```python
from build123d import *

# Parameters (mm, degrees)
MODEL_R             = 1.775
MODEL_R_2           = 1.575
MODEL_W             = 19.75
MODEL_H             = 93.75
MODEL_W_2           = 17.75
BOSS_EXTRUDE1_DEPTH = 10


with BuildPart() as part:
    # Model → Boss-Extrude1 (new body)
    with BuildSketch(Plane.XY):
        Polygon((57.946480534, -88.339102909), (57.946480534, -68.089102909), (54.771480534, -68.089102909), (54.771480534, -48.339102909), (57.946480534, -48.339102909), (57.946480534, -28.089102909), (54.771480534, -28.089102909), (54.771480534, -8.339102909), (57.946480534, -8.339102909), (57.946480534, 11.910897091), (54.771480534, 11.910897091), (54.771480534, 31.660897091), (57.946480534, 31.660897091), (57.946480534, 51.910897091), (54.771480534, 51.910897091), (54.771480534, 71.660897091), (57.946480534, 71.660897091), (57.946480534, 91.910897091), (54.771480534, 91.910897091), (54.771480534, 111.660897091), (57.946480534, 111.660897091), (57.946480534, 131.910897091), (54.771480534, 131.910897091), (54.771480534, 151.660897091), (57.946480534, 151.660897091), (57.946480534, 161.910897091), (-172.303519466, 161.910897091), (-172.303519466, 151.660897091), (-169.128519466, 151.660897091), (-169.128519466, 131.910897091), (-172.303519466, 131.910897091), (-172.303519466, 111.660897091), (-169.128519466, 111.660897091), (-169.128519466, 91.910897091), (-172.303519466, 91.910897091), (-172.303519466, 71.660897091), (-169.128519466, 71.660897091), (-169.128519466, 51.910897091), (-172.303519466, 51.910897091), (-172.303519466, 31.660897091), (-169.128519466, 31.660897091), (-169.128519466, 11.910897091), (-172.303519466, 11.910897091), (-172.303519466, -8.339102909), (-169.128519466, -8.339102909), (-169.128519466, -28.089102909), (-172.303519466, -28.089102909), (-172.303519466, -48.339102909), (-169.128519466, -48.339102909), (-169.128519466, -68.089102909), (-172.303519466, -68.089102909), (-172.303519466, -88.339102909), align=None)
        with Locations((-12.413986694, 38.429929163)):
            Circle(MODEL_R, mode=Mode.SUBTRACT)
        with Locations((4.096306466, 38.429929163)):
            Circle(MODEL_R_2, mode=Mode.SUBTRACT)
        with Locations((4.008638821, 82.124992621)):
            Circle(MODEL_R_2, mode=Mode.SUBTRACT)
        with Locations((-45.560089874, 82.12499262)):
            Circle(MODEL_R_2, mode=Mode.SUBTRACT)
        with Locations((-45.560089874, 38.429929163)):
            Circle(MODEL_R_2, mode=Mode.SUBTRACT)
        with Locations((-68.972284348, 38.429929163)):
            Circle(MODEL_R_2, mode=Mode.SUBTRACT)
        with Locations((-68.972284348, 82.12499262)):
            Circle(MODEL_R_2, mode=Mode.SUBTRACT)
        with Locations((-102.118387528, 38.429929163)):
            Circle(MODEL_R, mode=Mode.SUBTRACT)
        with Locations((-118.541013043, 38.429929163)):
            Circle(MODEL_R_2, mode=Mode.SUBTRACT)
        with Locations((-118.541013043, 82.12499262)):
            Circle(MODEL_R_2, mode=Mode.SUBTRACT)
        with Locations((-118.541013043, 116.547553094)):
            Circle(MODEL_R_2, mode=Mode.SUBTRACT)
        with Locations((-102.118387528, 128.129929163)):
            Circle(MODEL_R, mode=Mode.SUBTRACT)
        with Locations((-12.413986694, 128.129929163)):
            Circle(MODEL_R, mode=Mode.SUBTRACT)
        with Locations((4.008638821, 116.547553094)):
            Circle(MODEL_R_2, mode=Mode.SUBTRACT)
        with Locations((-142.266187111, 104.785897091)):
            Rectangle(MODEL_W, MODEL_H, mode=Mode.SUBTRACT)
        with Locations((26.821480534, 104.785897091)):
            Rectangle(MODEL_W_2, MODEL_H, mode=Mode.SUBTRACT)
    extrude(amount=BOSS_EXTRUDE1_DEPTH)


solid = part.part
```
Here's how the part is built. I have some questions about the finished solid (model axes, mm). A direction names the side the tool comes from. Round coordinates to 2 decimals unless told otherwise and drop trailing zeros. Loops run counter-clockwise (first coordinate to the right, second up) from the corner with the lowest first, then second, coordinate; pieces in that order, holes last. Notation, with made-up numbers: (87, 19) -> (139, 19) arc R11 cw to (139, 38) -> close; hole circle Ø3 at (-19, 27.5). An arc over 180 degrees is marked (long way). Answer as CSV lines item,"result". Start each with the question number.
1. For faces 4 (the face through (-169.129, -58, 5)), 5 (the face through (57.946, 122, 5)), 6 (the face through (17.946, 104, 5)), 7 (the face through (54.771, 142, 5)), which set-ups out of +Z, -Z, +X, -X, +Y, -Y let a thin tool reach every point of the face, with its end or its side?
2. I need wall thicknesses on probe 1 along X at (y, z) = (60, 2); probe 2 along X at (y, z) = (76, 6.5); probe 3 along Y at (x, z) = (-47, 4.25). Which ranges of each line are inside material? Lowest first, please. Write a range as from..to.
3. Imagine slicing it at A-A on y = 87. Write out the boundary of the cut face in (x, z), plus the area to 3 significant figures.
4. Imagine slicing it at D-D on y = 26. Write out the boundary of the cut face in (x, z).
5. I'm going to push flat-ended pins straight in: P1, Ø3, axis at x = -12.41, y = 128.13, coming from the -Z side; P2, Ø3, axis at y = 94.5, z = 4, coming from the -X side. Where does each tip first touch, or does it pass through?
6. Imagine slicing it at C-C on z = 8.25. State how many separate pieces and enclosed holes the cut face has, plus the area to 3 significant figures.
7. Imagine slicing it at B-B on y = 139. Write out the boundary of the cut face in (x, z).
8. If we mould it in two halves opening along X, with no side actions, what happens to faces 1 (the face through (27, 57.911, 5)), 2 (the face through (54.771, -18, 5)), 3 (the face through (-172.304, 2, 5))? For each: pulls with the +X half, pulls with the -X half, needs draft (parallel to the pull), parting line crosses it, or undercut.
Solution:
1,face 4,"+Z, -Z, -X"
1,face 5,"+Z, -Z, +X, +Y, -Y"
1,face 6,"+Z, -Z"
1,face 7,"+Z, -Z, +X"
2,probe 1,"-169.13..-152.14, -132.39..17.95, 35.7..54.77"
2,probe 2,"-172.3..-152.14, -132.39..17.95, 35.7..57.95"
2,probe 3,"-88.34..37.79, 39.07..81.49, 82.76..161.91"
3,outline,"(-172.3, 0) -> (-152.14, 0) -> (-152.14, 10) -> (-172.3, 10) -> close; (-132.39, 0) -> (17.95, 0) -> (17.95, 10) -> (-132.39, 10) -> close; (35.7, 0) -> (57.95, 0) -> (57.95, 10) -> (35.7, 10) -> close"
3,area,"1,930 mm²"
4,outline,"(-169.13, 0) -> (54.77, 0) -> (54.77, 10) -> (-169.13, 10) -> close"
5,P1,"through"
5,P2,"x = -169.13"
6,separate pieces,"1"
6,enclosed holes,"16"
6,area,"53,200 mm²"
7,outline,"(-169.13, 0) -> (-152.14, 0) -> (-152.14, 10) -> (-169.13, 10) -> close; (-132.39, 0) -> (17.95, 0) -> (17.95, 10) -> (-132.39, 10) -> close; (35.7, 0) -> (54.77, 0) -> (54.77, 10) -> (35.7, 10) -> close"
8,face 1,"undercut"
8,face 2,"pulls with the +X half"
8,face 3,"pulls with the -X half"
